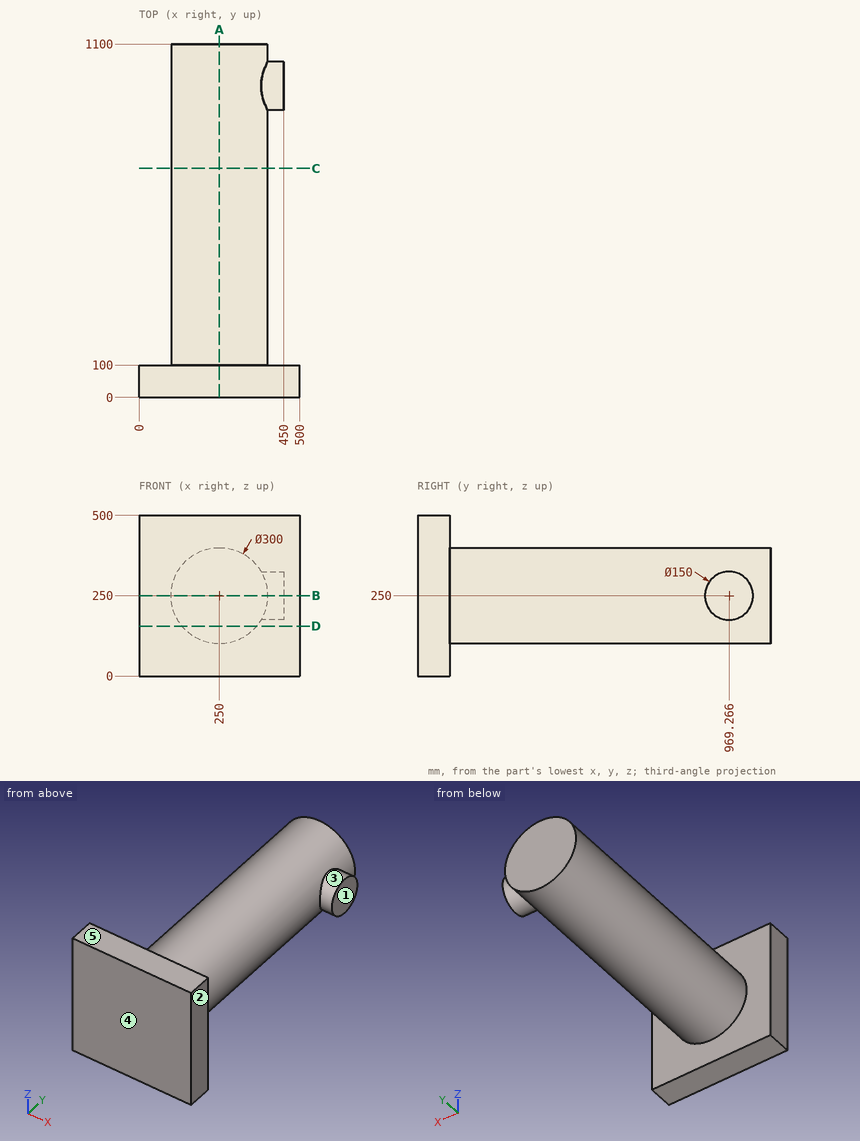
For this review, use the dimensioned drawing (mm, ordinates from the lowest corner) and the shaded views. A direction names the side the tool comes from. Coordinates: 2 decimals unless noted, no trailing zeros. Order: outer loops, then holes, each group sorted by start corner. A loop starts at its lowest first (then second) coordinate and runs counter-clockwise, first axis right, second up. Notation, with made-up numbers: (-25, 17.5) - (14, 17.5) arc R23 ccw to (14, 47.5) - close; hole circle Ø11 at (38.5, 72.25). An arc over 180 degrees is marked (long way). Answer as a JSON object with one key per item and string values. Group by question number.
1. For the marked faces 1 and 2, list the 3-axis set-ups (+Z, -Z, +X, -X, +Y, -Y) from which the entire face can be reached by the end or side of a thin tool; tool diameter is ignored.
2. We need section B-B on z = 250. State the section outline as (x, y) points (1 decimal).
3. We need section A-A on x = 250. State the section outline as (y, z) points.
4. Clearance check with flat-ended pins moving along their axes: P1, Ø6, axis at y = 455.5, z = 276, coming from the +X side; P2, Ø3, axis at x = 170, z = 447, coming from the +Y side; P3, Ø1, axis at x = 176, y = 856, coming from the +Z side. State where each tip first meets the part, or that it passes through.
5. We need section C-C on y = 712.5. State the section outline as (x, z) points, then the cut area to 3 significant figures.
6. For probe 1 along Y at (x, z) = (469.5, 108); probe 2 along Z at (x, y) = (255.5, 108.5); probe 3 along Y at (x, z) = (392.5, 187), list the stretches that pass through material, from the lowest coordinate up.
7. We need section D-D on z = 155. State the section outline as (x, y) points, then the cut area to 3 significant figures.
8. The part is to be moulded in two halves that separate along Y. For the marked faces 3, 4 and 5, say which applies: pulls with the +Y half, pulls with the -Y half, needs draft (parallel to the pull), parting line crosses it, or undercut.
Final values:
{
 "1": {"face 1": "+Z, -Z, +X, +Y", "face 2": "+Z, -Z, +X, +Y, -Y"},
 "2": {"outline": "(0, 0) - (500, 0) - (500, 100) - (400, 100) - (400, 894.3) - (450, 894.3) - (450, 1044.3) - (400, 1044.3) - (400, 1100) - (100, 1100) - (100, 100) - (0, 100) - close"},
 "3": {"outline": "(0, 0) - (100, 0) - (100, 100) - (1100, 100) - (1100, 400) - (100, 400) - (100, 500) - (0, 500) - close"},
 "4": {"P1": "x = 398.23", "P2": "y = 100", "P3": "z = 380.76"},
 "5": {"outline": "circle Ø300 at (250, 250)", "area": "70,700 mm²"},
 "6": {"probe 1": "0 to 100", "probe 2": "100.1 to 399.9", "probe 3": "0 to 100, 928.57 to 1009.96"},
 "7": {"outline": "(0, 0) - (500, 0) - (500, 100) - (366.08, 100) - (366.08, 1100) - (133.92, 1100) - (133.92, 100) - (0, 100) - close", "area": "282,000 mm²"},
 "8": {"face 3": "undercut", "face 4": "pulls with the -Y half", "face 5": "needs draft"}
}
